```python
from build123d import *

# Parameters (mm, degrees)
BOSS_EXTRUDE1_DEPTH = 7.5
CUT_EXTRUDE1_DEPTH  = 2
BOSS_EXTRUDE2_DEPTH = 2
CUT_EXTRUDE2_DEPTH  = 15
SKETCH6_W           = 1
SKETCH6_H           = 1
CUT_EXTRUDE3_DEPTH  = 2
SKETCH7_W           = 0.5
SKETCH7_H           = 0.5
CUT_EXTRUDE4_DEPTH  = 1


with BuildPart() as part:
    # Sketch1 → Boss-Extrude1 (new body)
    # profile 1 of 2: a face of its own
    with BuildSketch(Plane(origin=(0, 0, 0), x_dir=(1, 0, 0), z_dir=(0, 1, 0))):
        Polygon((-5.196152423, -9), (5.196152423, -9), (10.392304845, 0), (5.196152423, 9), (-5.196152423, 9), (-10.392304845, 0), align=None)
        Polygon((4.330127019, -7.5), (8.660254038, 0), (4.330127019, 7.5), (-4.330127019, 7.5), (-8.660254038, 0), (-4.330127019, -7.5), align=None, mode=Mode.SUBTRACT)
    # profile 2 of 2: a face of its own
    with BuildSketch(Plane(origin=(0, 0, 0), x_dir=(1, 0, 0), z_dir=(0, 1, 0))):
        Polygon((-4.330127019, -7.5), (4.330127019, -7.5), (8.660254038, 0), (4.330127019, 7.5), (-4.330127019, 7.5), (-8.660254038, 0), align=None)
    extrude(amount=BOSS_EXTRUDE1_DEPTH)

    # Sketch1<3> → Cut-Extrude1 (cut)
    with BuildSketch(Plane(origin=(0, 0, 0), x_dir=(1, 0, 0), z_dir=(0, 1, 0))):
        Polygon((-4.330127019, -7.5), (4.330127019, -7.5), (8.660254038, 0), (4.330127019, 7.5), (-4.330127019, 7.5), (-8.660254038, 0), align=None)
    extrude(amount=CUT_EXTRUDE1_DEPTH, mode=Mode.SUBTRACT)

    # Sketch4 → Boss-Extrude2 (add)
    with BuildSketch(Plane(origin=(0, 7.5, 0), x_dir=(1, 0, 0), z_dir=(0, 1, 0))):
        Polygon((8.660254038, 0), (4.330127019, 7.5), (-4.330127019, 7.5), (-8.660254038, 0), (-4.330127019, -7.5), (4.330127019, -7.5), align=None)
    extrude(amount=BOSS_EXTRUDE2_DEPTH)

    # Sketch5 → Cut-Extrude2 (cut)
    with BuildSketch(Plane(origin=(-6.495190528, 0, 3.75), x_dir=(0.5000000000000006, 0, 0.8660254037844384), z_dir=(-0.8660254037844384, 0, 0.5000000000000006))):
        with BuildLine():
            ThreePointArc((-3.080127019, 8.25), (-2.860457105, 7.719669914), (-2.330127019, 7.5))
            Line((-2.330127019, 7.5), (2.330127019, 7.5))
            ThreePointArc((2.330127019, 7.5), (2.860457105, 7.719669914), (3.080127019, 8.25))
            ThreePointArc((3.080127019, 8.25), (3.446243542, 9.133883476), (4.330127019, 9.5))
            Line((4.330127019, 9.5), (-4.330127019, 9.5))
            ThreePointArc((-4.330127019, 9.5), (-3.446243542, 9.133883476), (-3.080127019, 8.25))
        make_face()
    extrude(amount=-CUT_EXTRUDE2_DEPTH, mode=Mode.SUBTRACT)

    # Sketch6 → Cut-Extrude3 (cut)
    with BuildSketch(Plane(origin=(-7.794228634, 0, 4.5), x_dir=(0.5000000000000071, 0, 0.8660254037844346), z_dir=(-0.8660254037844345, 0, 0.500000000000007))):
        with Locations((-3.830127019, 4.273741672)):
            Rectangle(SKETCH6_W, SKETCH6_H)
    cut_extrude3 = extrude(amount=-CUT_EXTRUDE3_DEPTH, mode=Mode.SUBTRACT)

    # Sketch7 → Cut-Extrude4 (cut)
    with BuildSketch(Plane(origin=(-2.165063509, 0, -3.75), x_dir=(0.8660254037844346, 0, -0.5000000000000071), z_dir=(0.5000000000000071, 0, 0.8660254037844346))):
        with Locations((-7.25, 3.523741672)):
            Rectangle(SKETCH7_W, SKETCH7_H)
    cut_extrude4 = extrude(amount=CUT_EXTRUDE4_DEPTH, mode=Mode.SUBTRACT)

    # Mirror1: Cut-Extrude3, Cut-Extrude4 across plane
    add(cut_extrude3.mirror(Plane(origin=(0, 0, 0), x_dir=(-0.8660254037844349, 0, 0.5000000000000067), z_dir=(-0.500000000000007, 0, -0.8660254037844347))), mode=Mode.SUBTRACT)
    add(cut_extrude4.mirror(Plane(origin=(0, 0, 0), x_dir=(-0.8660254037844349, 0, 0.5000000000000067), z_dir=(-0.500000000000007, 0, -0.8660254037844347))), mode=Mode.SUBTRACT)


solid = part.part
```
Model file for the job. Use its own axes, mm. A direction names the side the tool comes from. Coordinates: 2 decimals unless noted, no trailing zeros. Loops run counter-clockwise (first coordinate to the right, second up) from the corner with the lowest first, then second, coordinate; pieces in that order, holes last. Notation, with made-up numbers: (50.5, -37) -> (63.5, -37) arc R16 cw to (63.5, -26) -> close; hole circle Ø8 at (48.25, 84). An arc over 180 degrees is marked (long way). Answer as a JSON object with one key per item and string values.
Q1. Cut at A-A (y = 1.75). List the corners of the cut face in (x, z).
Report:
{"outline": "(-10.39, 0) -> (-5.2, -9) -> (5.2, -9) -> (10.39, 0) -> (5.2, 9) -> (-5.2, 9) -> close; hole (-8.66, 0) -> (-4.33, -7.5) -> (4.33, -7.5) -> (8.66, 0) -> (4.33, 7.5) -> (-4.33, 7.5) -> close"}
Q2. Cut at C-C (y = 8). List the corners of the cut face in (x, z).
Report:
{"outline": "(-8.66, 0) -> (-4.33, -7.5) -> (4.33, -7.5) -> (4.98, -6.38) -> (-8.01, 1.12) -> close; (-4.98, 6.38) -> (8.01, -1.12) -> (8.66, 0) -> (4.33, 7.5) -> (-4.33, 7.5) -> close"}
Q3. Flat gauge pins, fed straight in: P1, Ø6, axis at x = 7, z = -4.5, coming from the +Y side; P2, Ø1.3, axis at x = -9, z = 1, coming from the +Y side; P3, Ø3, axis at x = -5, z = -2, coming from the -Y side. Where does each tip first touch, or does it go through?
Report:
{"P1": "stops at y = 8.94", "P2": "stops at y = 7.5", "P3": "stops at y = 2"}
Q4. Pull direction X, two halves, no side cores. Call faces 5 (the flat face through (0, 1, 7.5)), 6 (the flat face through (-7.76, 3.7, -4.56)), 7 (the flat face through (3, 9.5, 5)): released by +X, released by -X, zero draft, split by the parting line, or undercut.
Report:
{"face 5": "undercut", "face 6": "released by -X", "face 7": "zero draft"}
Q5. Cut at B-B (x = -9). List the corners of the cut face in (y, z), and give its area (3 significant figures).
Report:
{"outline": "(0, -2.41) -> (7.5, -2.41) -> (7.5, 2.41) -> (0, 2.41) -> close; hole (3.77, 0.2) -> (4.77, 0.2) -> (4.77, 1.35) -> (3.77, 1.35) -> close", "area": "35.0 mm2"}
Q6. 3-axis set-ups, long thin cutter, end or side, ignore diameter. For faces 1 (the flat face through (-4.615, 8.264, 7.007)), 2 (the flat face through (-4.144, 4.034, 6.823)), 3 (the flat face through (-6.465, 0.986, -3.802)), 4 (the flat face through (-6.465, 8.486, -3.802)): which of +Z, -Z, +X, -X, +Y, -Y reach the whole face in a straight line?
Report:
{"face 1": "+Z, -X, +Y", "face 2": "none", "face 3": "-Y", "face 4": "-Z, -X, +Y"}
Q7. Probe probe 1 along Y at (x, z) = (-7.75, -1.5); probe 2 along Y at (x, z) = (8.5, -0.5); probe 3 along X at (y, z) = (1.5, 1.5). List the from-to ranges inside material, lowest first.
Report:
{"probe 1": "y = 2 to 9.5", "probe 2": "y = 0 to 7.5", "probe 3": "x = -9.53 to -7.79, 7.79 to 9.53"}
